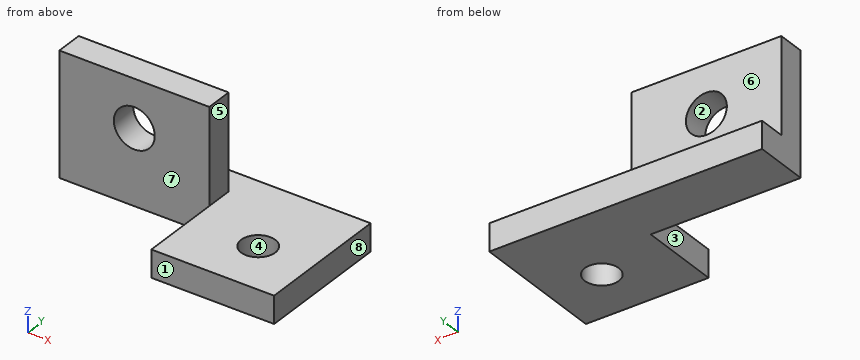
from build123d import *

# Parameters (mm, degrees)
F0_R     = 3.9751
F1_DEPTH = 3.175
F2_W     = 34.925
F2_H     = 22.225
F2_R     = 4.7625
F3_DEPTH = 6.35


with BuildPart() as f1:
    # F0 (on Top) → F1 (new body, symmetric)
    with BuildSketch(Plane.XY):
        Polygon((0, 19.05), (0, 0), (28.575, 0), (28.575, 31.75), (-34.925, 31.75), (-34.925, 19.05), align=None)
        with Locations((15.875, 12.7)):
            Circle(F0_R, mode=Mode.SUBTRACT)
    extrude(amount=F1_DEPTH, both=True)

    # F2 (on face) → F3 (join)
    with BuildSketch(Plane.XZ.offset(-19.05)):
        with Locations((-17.4625, 14.2875)):
            Rectangle(F2_W, F2_H)
        with Locations((-17.4625, 14.2875)):
            Circle(F2_R, mode=Mode.SUBTRACT)
    extrude(amount=-F3_DEPTH)


solid = f1.part
Verification items for the finished model (mm, model axes). Face numbers are marked on the shaded views. A direction names the side the tool comes from. Coordinates: 2 decimals unless noted, no trailing zeros. Write each loop counter-clockwise with the first axis right and the second up, starting at its lowest first coordinate (ties: lowest second). Pieces come first, ordered by that corner, then holes. Notation, with made-up numbers: M 1,9.5 L 15,9.5 A35 ccw 15,47.5 Z; hole C 88.25,-31 d7. An arc over 180 degrees is marked long. Use a Markdown table: item, result.
Q1. Sectioned sample at D-D, the plane x = -9. Record the boundary of the cut face in (y, z) (3 decimals).
Reply:
| item | result |
|---|---|
| outline | M 19.05,-3.175 L 31.75,-3.175 L 31.75,3.175 L 25.4,3.175 L 25.4,25.4 L 19.05,25.4 Z |
Q2. Sectioned sample at C-C, the plane x = -17. Record the boundary of the cut face in (y, z) (3 decimals).
Reply:
| item | result |
|---|---|
| outline | M 19.05,-3.175 L 31.75,-3.175 L 31.75,3.175 L 25.4,3.175 L 25.4,9.548 L 19.05,9.548 Z; M 19.05,19.027 L 25.4,19.027 L 25.4,25.4 L 19.05,25.4 Z |
Q3. Thickness scan on line 1 (Y direction, x = -4.5, z = 20.75); line 2 (Z direction, x = -22.5, y = 27) (3 decimals); line 3 (Y direction, x = 13, z = 2.5). Record the ranges inside material, lowest first.
Reply:
| item | result |
|---|---|
| line 1 | y = 19.05 to 25.4 |
| line 2 | z = -3.175 to 3.175 |
| line 3 | y = 0 to 9.95, 15.45 to 31.75 |
Q4. Set-up check for the marked faces 4, 5, 6, 7 and 8: record each of +Z, -Z, +X, -X, +Y, -Y from which the full face is reachable in a straight line by a thin tool's end or side.
Reply:
| item | result |
|---|---|
| face 4 | +Z, -Z |
| face 5 | +Z, +X, +Y, -Y |
| face 6 | +Z, +X, -X, +Y |
| face 7 | +Z, -Z, -X, -Y |
| face 8 | +Z, -Z, +X, +Y, -Y |
Q5. Sectioned sample at A-A, the plane y = 12.7. Record the boundary of the cut face in (x, z) (3 decimals).
Reply:
| item | result |
|---|---|
| outline | M 0,-3.175 L 11.9,-3.175 L 11.9,3.175 L 0,3.175 Z; M 19.85,-3.175 L 28.575,-3.175 L 28.575,3.175 L 19.85,3.175 Z |
Q6. Sectioned sample at B-B, the plane z = 0.5. Record the boundary of the cut face in (x, y) (3 decimals), plus the area to 3 significant figures.
Reply:
| item | result |
|---|---|
| outline | M -34.925,19.05 L 0,19.05 L 0,0 L 28.575,0 L 28.575,31.75 L -34.925,31.75 Z; hole C 15.875,12.7 d7.95 |
| area | 1,300 mm² |
Q7. Go/stop test with flat-tipped pins: P1, Ø12, axis at x = -17, z = 9.5, coming from the -Y side; P2, Ø15, axis at x = -17.46, z = 14.29, coming from the +Y side; P3, Ø12.5, axis at x = 15.875, y = 12.7, coming from the +Z side (3 decimals). Record where each tip stops, or that it passes through.
Reply:
| item | result |
|---|---|
| P1 | stops at y = 19.05 |
| P2 | stops at y = 25.4 |
| P3 | stops at z = 3.175 |
Q8. Draft check along X on the marked faces 1, 2 and 3. Enter one of: +X half, -X half, draft (parallel to the pull), parting line (faces both ways), or undercut.
Reply:
| item | result |
|---|---|
| face 1 | draft |
| face 2 | undercut |
| face 3 | -X half |
